from build123d import *
from build123d.topology import SkipClean

# Parameters (mm, degrees)
SKETCH_1_W          = 46.6
SKETCH_1_H          = 7.3
EXTRUDE_1_DEPTH     = 54
EXTRUDE_1_2_DEPTH   = 54
SKETCH_2_W          = 46.6
SKETCH_2_H          = 45.4
EXTRUDE_2_DEPTH     = 4
SKETCH_3_W          = 54
SKETCH_3_H          = 60
EXTRUDE_3_DEPTH     = 3
SKETCH_4_R          = 3.871689423
CUT_EXTRUDE_1_DEPTH = 3
EXTRUDE_4_DEPTH     = 75
SKETCH_6_W          = 75
SKETCH_6_H          = 7.3
EXTRUDE_5_DEPTH     = 27.146082
SKETCH_7_W          = 4
SKETCH_7_H          = 60
EXTRUDE_6_DEPTH     = 104.5
SKETCH_8_R          = 1.4
CUT_EXTRUDE_2_DEPTH = 75
SKETCH_10_W         = 104.5
SKETCH_10_H         = 50
EXTRUDE_7_DEPTH     = 7.3
SKETCH_11_R         = 7.5
SKETCH_11_R_2       = 5
CUT_EXTRUDE_3_DEPTH = 16
SKETCH_12_W         = 54
SKETCH_12_H         = 60
EXTRUDE_8_DEPTH     = 3
SKETCH_13_R         = 1.4
CUT_EXTRUDE_4_DEPTH = 15
FILLET_1_R          = 2
FILLET_2_R          = 2


with BuildPart() as part:
    # Sketch 1 → Extrude 1 (new body)
    with BuildSketch(Plane.XY):
        with Locations((26.3, 3.65)):
            Rectangle(SKETCH_1_W, SKETCH_1_H)
    extrude(amount=EXTRUDE_1_DEPTH)



with BuildPart() as body_2:
    # Sketch 1 → Extrude 1 2 (new body)
    with BuildSketch(Plane.XY):
        with Locations((26.3, 56.35)):
            Rectangle(SKETCH_1_W, SKETCH_1_H)
    extrude(amount=EXTRUDE_1_2_DEPTH)


with BuildPart() as part_1:
    add(part.part)

    add(body_2.part)  # Extrude 2 merges body 2
    # Sketch 2 → Extrude 2 (add)
    with BuildSketch(Plane(origin=(0, 0, 0), x_dir=(-1, 0, 0), z_dir=(0, 0, -1))):
        with Locations((-26.3, 30)):
            Rectangle(SKETCH_2_W, SKETCH_2_H)
    extrude(amount=-EXTRUDE_2_DEPTH)

    # Sketch 3 → Extrude 3 (add)
    with BuildSketch(Plane.ZY.offset(-3)):
        with Locations((27, 30)):
            Rectangle(SKETCH_3_W, SKETCH_3_H)
    extrude(amount=EXTRUDE_3_DEPTH)

    # Sketch 4 → Cut-Extrude 1 (cut)
    with BuildSketch(Plane(origin=(3, 0, 0), x_dir=(0, 0, -1), z_dir=(1, 0, 0))):
        with Locations((-26.853917863, 29.837440161)):
            Circle(SKETCH_4_R)
    extrude(amount=-CUT_EXTRUDE_1_DEPTH, mode=Mode.SUBTRACT)

    # Sketch 5 → Extrude 4 (add)
    with BuildSketch(Plane(origin=(49.6, 0, 0), x_dir=(0, 0, -1), z_dir=(1, 0, 0))):
        Polygon((0, 0), (0, 60), (-26.853917863, 60), (-26.853917863, 52.7), (-4, 52.7), (-4, 7.3), (-26.853917863, 7.3), (-26.853917863, 0), align=None)
        with BuildLine():
            Line((-4, 52.7), (-26.853917863, 52.7))
            Line((-26.853917863, 52.7), (-26.853917863, 47.837440161))
            ThreePointArc((-26.853917863, 47.837440161), (-14.125995802, 42.565362223), (-8.853917863, 29.837440161))
            ThreePointArc((-8.853917863, 29.837440161), (-14.125995802, 17.1095181), (-26.853917863, 11.837440161))
            Line((-26.853917863, 11.837440161), (-26.853917863, 7.3))
            Line((-26.853917863, 7.3), (-4, 7.3))
            Line((-4, 7.3), (-4, 52.7))
        make_face()
    extrude(amount=EXTRUDE_4_DEPTH)

    # Sketch 6 → Extrude 5 (add)
    with BuildSketch(Plane.XY.offset(26.853917863)):
        with Locations((87.1, 56.35)):
            Rectangle(SKETCH_6_W, SKETCH_6_H)
        with Locations((87.1, 3.65)):
            Rectangle(SKETCH_6_W, SKETCH_6_H)
    extrude(amount=EXTRUDE_5_DEPTH)

    # Sketch 7 → Extrude 6 (add)
    with BuildSketch(Plane(origin=(124.6, 0, 0), x_dir=(0, 0, -1), z_dir=(1, 0, 0))):
        with Locations((-2, 30)):
            Rectangle(SKETCH_7_W, SKETCH_7_H)
    extrude(amount=EXTRUDE_6_DEPTH)

    # Sketch 8 → Cut-Extrude 2 (cut)
    with BuildSketch(Plane.XY.offset(4)):
        with Locations((147.6, 31)):
            Circle(SKETCH_8_R)
        with Locations((180.6, 45)):
            Circle(SKETCH_8_R)
        with Locations((186.6, 31)):
            Circle(SKETCH_8_R)
        with Locations((219.6, 45)):
            Circle(SKETCH_8_R)
    extrude(amount=-CUT_EXTRUDE_2_DEPTH, mode=Mode.SUBTRACT)

    # Sketch 10 → Extrude 7 (add)
    with SkipClean():  # the faces are left unmerged after this step: merging them gives an invalid solid
        with BuildSketch(Plane(origin=(0, 60, 0), x_dir=(1, 0, 0), z_dir=(0, 1, 0))):
            with Locations((176.85, -29)):
                Rectangle(SKETCH_10_W, SKETCH_10_H)
        extrude(amount=-EXTRUDE_7_DEPTH)

    # Sketch 11 → Cut-Extrude 3 (cut)
    with SkipClean():  # the faces are left unmerged after this step: merging them gives an invalid solid
        with BuildSketch(Plane(origin=(0, 52.7, 0), x_dir=(-1, 0, 0), z_dir=(0, -1, 0))):
            with Locations(Location((-164.1, -14, 0), (0, 0, 90))):
                Circle(SKETCH_11_R)
            with Locations(Location((-203.1, -14, 0), (0, 0, 90))):
                Circle(SKETCH_11_R)
            with Locations(Location((-199.075229873, -33.590845449, 0), (0, 0, 90))):
                Circle(SKETCH_11_R_2)
            with Locations(Location((-160.075229873, -33.590845449, 0), (0, 0, 90))):
                Circle(SKETCH_11_R_2)
        extrude(amount=-CUT_EXTRUDE_3_DEPTH, mode=Mode.SUBTRACT)

    # Sketch 12 → Extrude 8 (add)
    with BuildSketch(Plane(origin=(229.1, 0, 0), x_dir=(0, 0, -1), z_dir=(1, 0, 0))):
        with Locations((-27, 30)):
            Rectangle(SKETCH_12_W, SKETCH_12_H)
    extrude(amount=-EXTRUDE_8_DEPTH)

    # Sketch 13 → Cut-Extrude 4 (cut)
    with BuildSketch(Plane.XY.offset(54)):
        with Locations((3.5, 3.5)):
            Circle(SKETCH_13_R)
        with Locations((3.5, 56.5)):
            Circle(SKETCH_13_R)
        with Locations((225.6, 56.5)):
            Circle(SKETCH_13_R)
    extrude(amount=-CUT_EXTRUDE_4_DEPTH, mode=Mode.SUBTRACT)

    # Fillet 1
    fillet_1_edges = [part_1.edges().sort_by_distance(p)[0] for p in [
        (49.6, 29.837440161, 8.853917863),
        (49.6, 50.268720081, 26.853917863),
        (124.6, 29.837440161, 8.853917863),
        (87.1, 47.837440161, 26.853917863),
        (49.6, 9.568720081, 26.853917863),
        (87.1, 11.837440161, 26.853917863),
        (124.6, 9.568720081, 26.853917863),
        (124.6, 50.268720081, 26.853917863),
    ]]
    fillet(fillet_1_edges, radius=FILLET_1_R)

    # Fillet 2
    fillet_2_edges = [part_1.edges().sort_by_distance(p)[0] for p in [
        (229.1, 60, 27),
        (0, 60, 27),
    ]]
    fillet(fillet_2_edges, radius=FILLET_2_R)


solid = part_1.part
Verification items for the finished model (mm, model axes). A direction names the side the tool comes from. Coordinates: 2 decimals unless noted, no trailing zeros. Loops run counter-clockwise (first coordinate to the right, second up) from the corner with the lowest first, then second, coordinate; pieces in that order, holes last. Notation, with made-up numbers: (23.5, -27) -> (67.5, -27) arc R6 ccw to (67.5, -22) -> close; hole circle Ø2 at (41.5, 83). An arc over 180 degrees is marked (long way). Answer as a JSON object with one key per item and string values. Group by question number.
Item 1: Mould release check, pull along Y, two halves, no side actions. Record for faces 1 (the cylindrical face through (1.521, 26.058, 27.693)), 2 (the flat face through (0, 29, 33)), 3 (the flat face through (65, 0, 27)): +Y half, -Y half, draft (parallel to the pull), parting line (faces both ways), or undercut.
Item 2: Sectioned sample at B-B on z = 14. State how many separate pieces and enclosed holes the cut face has, plus the area to 3 significant figures.
Item 3: Scan lines: probe 1 along X at (y, z) = (54.75, 14); probe 2 along X at (y, z) = (13, 14.5); probe 3 along Y at (x, z) = (3.5, 47.25). Record each from-to range of solid material in increasing order.
Item 4: Depth check by flat-ended pin: pin 1 (16 mm diameter, centred on x = 166.5, y = 33.5, fed in from +Z); pin 2 (2 mm diameter, centred on x = 147.6, y = 31, fed in from -Z); pin 3 (0.8 mm diameter, centred on x = 4, y = 56, fed in from +Z). Enter the tip coordinate at first touch or a pass-through.
Item 5: Tool access check on faces 4 (the flat face through (49.6, 30, 5)), 5 (the cylindrical face through (165.033, 56.299, 34.242)), 6 (the flat face through (175, 26, 4)). Record the directions out of +Z, -Z, +X, -X, +Y, -Y that give a thin tool (end or side, any length) a straight path to the whole face; none if there is none.
Item 6: Sectioned sample at A-A on x = 99. Record the boundary of the cut face in (y, z), plus the area to 3 significant figures.
Evaluation:
{
 "1": {"face 1": "undercut", "face 2": "draft", "face 3": "-Y half"},
 "2": {"separate pieces": "3", "enclosed holes": "0", "area": "4,170 mm²"},
 "3": {"probe 1": "x = 0 to 156.6, 171.6 to 195.6, 210.6 to 229.1", "probe 2": "x = 0 to 3, 49.6 to 124.6, 226.1 to 229.1", "probe 3": "y = 0 to 2.1, 4.9 to 7.3, 52.7 to 55.1, 57.9 to 60"},
 "4": {"pin 1": "stops at z = 4", "pin 2": "passes through", "pin 3": "stops at z = 39"},
 "5": {"face 4": "+Z", "face 5": "+Y, -Y", "face 6": "+Z, -Y"},
 "6": {"outline": "(0, 0) -> (60, 0) -> (60, 54) -> (52.7, 54) -> (52.7, 26.85) -> (49.74, 26.85) arc R2 ccw to (47.75, 25.05) arc R18 cw to (11.93, 25.05) arc R2 ccw to (9.94, 26.85) -> (7.3, 26.85) -> (7.3, 54) -> (0, 54) -> close", "area": "1,500 mm²"}
}
